Here's how the part is built. I have some questions about the finished solid (model axes, mm). Round coordinates to 2 decimals unless told otherwise and drop trailing zeros. Order: outer loops, then holes, each group sorted by start corner. A loop starts at its lowest first (then second) coordinate and runs counter-clockwise, first axis right, second up. Notation, with made-up numbers: M -5.75,12 L 26.25,12 A11 ccw 26.25,18 Z; hole C 54,6 d4. An arc over 180 degrees is marked long. Write each question's results on one line, items separated by ' | '. Start each with the question number.
```python
from build123d import *

# Parameters (mm, degrees)
SKETCH1_R           = 1.375
BOSS_EXTRUDE1_DEPTH = 4
SKETCH3_R           = 1.5
SKETCH3_R_2         = 65
CUT_EXTRUDE1_DEPTH  = 145.688169592


with BuildPart() as part:
    # Sketch1 → Boss-Extrude1 (new body)
    with BuildSketch(Plane.XY):
        with BuildLine():
            ThreePointArc((-29.484078319, 77.051535518), (-71.447095812, 41.25), (-81.470626319, -12.991806928))
            ThreePointArc((-81.470626319, -12.991806928), (-83.101535217, -32.169647267), (-93.500519111, -48.365651648))
            ThreePointArc((-93.500519111, -48.365651648), (-94.396769013, -54.5), (-88.636142553, -56.790998993))
            ThreePointArc((-88.636142553, -56.790998993), (-69.410499373, -55.883216958), (-51.986548, -64.05972859))
            ThreePointArc((-51.986548, -64.05972859), (0, -82.5), (51.986548, -64.05972859))
            ThreePointArc((51.986548, -64.05972859), (69.410499373, -55.883216958), (88.636142553, -56.790998993))
            ThreePointArc((88.636142553, -56.790998993), (94.396769013, -54.5), (93.500519111, -48.365651648))
            ThreePointArc((93.500519111, -48.365651648), (83.101535217, -32.169647267), (81.470626319, -12.991806928))
            ThreePointArc((81.470626319, -12.991806928), (71.447095812, 41.25), (29.484078319, 77.051535518))
            ThreePointArc((29.484078319, 77.051535518), (13.691035844, 88.052864225), (4.864376558, 105.156650641))
            ThreePointArc((4.864376558, 105.156650641), (0, 109), (-4.864376558, 105.156650641))
            ThreePointArc((-4.864376558, 105.156650641), (-13.691035844, 88.052864225), (-29.484078319, 77.051535518))
        make_face()
        with Locations((0, 104)):
            Circle(SKETCH1_R, mode=Mode.SUBTRACT)
        with Locations((90.066641994, -52)):
            Circle(SKETCH1_R, mode=Mode.SUBTRACT)
        with Locations((-90.066641994, -52)):
            Circle(SKETCH1_R, mode=Mode.SUBTRACT)
    extrude(amount=BOSS_EXTRUDE1_DEPTH)

    # Sketch3 → Cut-Extrude1 (cut, through all)
    with BuildSketch(Plane.XY.offset(4)):
        with Locations((0, 74)):
            Circle(SKETCH3_R)
        with Locations((-64.08587988, -37)):
            Circle(SKETCH3_R)
        with Locations((64.08587988, -37)):
            Circle(SKETCH3_R)
        with Locations((-64.08587988, 37)):
            Circle(SKETCH3_R)
        with Locations((64.08587988, 37)):
            Circle(SKETCH3_R)
        with Locations((0, -74)):
            Circle(SKETCH3_R)
        Circle(SKETCH3_R_2)
    extrude(amount=-CUT_EXTRUDE1_DEPTH, mode=Mode.SUBTRACT)


solid = part.part
```
(1) If we mould it in two halves opening along X, with no side actions, what happens to faces 1 (the cylindrical face through (13.87, 87.85, 1.97)), 2 (the cylindrical face through (62, 19.52, 2.03)), 3 (the flat face through (-43, 49, 0))? For each: pulls with the +X half, pulls with the -X half, needs draft (parallel to the pull), parting line crosses it, or undercut.
(2) I want a section at B-B on x = -25.5. Write out the boundary of the cut face in (y, z).
(3) I want a section at D-D on y = 83.5. Write out the boundary of the cut face in (x, z).
(4) I want a section at A-A on y = 0. Write out the boundary of the cut face in (x, z).
(5) I'm going to push flat-ended pins straight in: pin 1 Ø1 at (y, z) = (63.5, 3) entering from +X; pin 2 Ø2 at (x, z) = (-54, 3) entering from +Y; pin 3 Ø1 at (y, z) = (-9.5, 3) entering from +X. Where does each tip first touch, or does it pass through?
(6) I want a section at C-C on z = 0.8. Give the number of separate pieces and of enclosed holes in the cut face, and give its area (3 significant figures).
(7) Please list where these lines run through material, in increasing order: line 1 (Y direction, x = 54.5, z = 1.9); line 2 (X direction, y = -74, z = 2.55); line 3 (Y direction, x = -49, z = 2.2).
Solutions:
1) face 1: pulls with the +X half | face 2: undercut | face 3: needs draft
2) outline: M -78.46,0 L -59.79,0 L -59.79,4 L -78.46,4 Z; M 59.79,0 L 78.83,0 L 78.83,4 L 59.79,4 Z
3) outline: M -18.39,0 L 18.39,0 L 18.39,4 L -18.39,4 Z
4) outline: M -82.5,0 L -65,0 L -65,4 L -82.5,4 Z; M 65,0 L 82.5,0 L 82.5,4 L 65,4 Z
5) pin 1: x = 53.27 | pin 2: y = 63.22 | pin 3: x = 82.01
6) separate pieces: 1 | enclosed holes: 10 | area: 9,680 mm^2
7) line 1: -62.18 to -35.42, 35.42 to 61.94 | line 2: -36.47 to -1.5, 1.5 to 36.47 | line 3: -66.37 to -42.71, 42.71 to 66.37
